Source: three-view drawing plus pictorial views. Frame: mm from the lowest corner of the part. Give positions to 0.01 mm unless a question says otherwise; leave off trailing zeros. Write each loop counter-clockwise with the first axis right and the second up, starting at its lowest first coordinate (ties: lowest second). Pieces come first, ordered by that corner, then holes.
Q1. Cut plane C-C on x = 43.4. Return the cut outline in (y, z).
Q2. Cut plane B-B on x = 60. Return the cut outline in (y, z), plus the area to 3 significant figures.
Q3. Line query: L1, parallel to X at y = 65.5, z = 3.1; L2, parallel to Y at x = 92.4, z = 1.9; L3, parallel to Y at x = 43.4, z = 2. Output: solid intervals per line, ascending.
Q4. Cut plane A-A on y = 60. Return the cut outline in (x, z).
Q5. Cut plane D-D on z = 3.05. Count the separate pieces of the cut face and the enclosed holes in it, plus the area to 3 significant figures.
Q6. Pin query (flat end, axial travel): pin 1 (3 mm diameter, centred on y = 64.5, z = 3, fed in from +X); pin 2 (2.5 mm diameter, centred on x = 24.645, y = 24.645, fed in from +Z) (3 decimals); pin 3 (1.7 mm diameter, centred on x = 62, z = 4, fed in from +Y). Return the tip coordinate at first contact, or that it passes through.
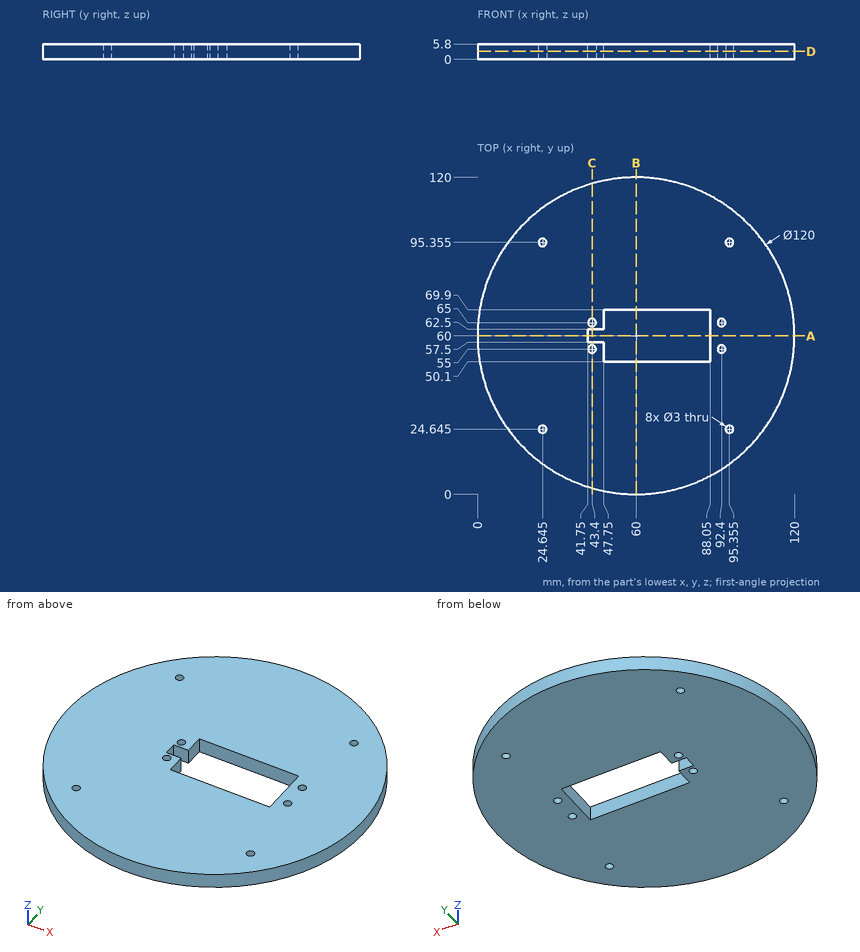
Data:
1. outline: (2.34, 0) - (53.5, 0) - (53.5, 5.8) - (2.34, 5.8) - close; (56.5, 0) - (57.5, 0) - (57.5, 5.8) - (56.5, 5.8) - close; (62.5, 0) - (63.5, 0) - (63.5, 5.8) - (62.5, 5.8) - close; (66.5, 0) - (117.66, 0) - (117.66, 5.8) - (66.5, 5.8) - close
2. outline: (0, 0) - (50.1, 0) - (50.1, 5.8) - (0, 5.8) - close; (69.9, 0) - (120, 0) - (120, 5.8) - (69.9, 5.8) - close
2. area: 581 mm2
3. L1: x = 0.25 to 41.99, 44.81 to 47.75, 88.05 to 90.99, 93.81 to 119.75
3. L2: y = 9.5 to 53.5, 56.5 to 63.5, 66.5 to 110.5
3. L3: y = 2.34 to 53.5, 56.5 to 57.5, 62.5 to 63.5, 66.5 to 117.66
4. outline: (0, 0) - (41.75, 0) - (41.75, 5.8) - (0, 5.8) - close; (88.05, 0) - (120, 0) - (120, 5.8) - (88.05, 5.8) - close
5. separate pieces: 1
5. enclosed holes: 9
5. area: 10,400 mm2
6. pin 1: stops at x = 119.92
6. pin 2: passes through
6. pin 3: stops at y = 119.99
